The listing builds one solid part. Answer for the finished solid, in the listing's coordinates (mm). A direction names the side the tool comes from. Give positions to 0.01 mm unless a question says otherwise; leave off trailing zeros. Loops run counter-clockwise (first coordinate to the right, second up) from the corner with the lowest first, then second, coordinate; pieces in that order, holes last. Notation, with made-up numbers: M -4.5,74 L 0.5,74 A21 ccw 0.5,86 Z; hole C 30.25,-23.5 d4. An arc over 180 degrees is marked long. Return JSON: item names as keys, results as strings.
from build123d import *

# Parameters (mm, degrees)
SKETCH_1_W          = 400
SKETCH_1_H          = 350
EXTRUDE_1_DEPTH     = 80
SKETCH_2_W          = 394
SKETCH_2_H          = 344
EXTRUDE_2_DEPTH     = 10
SKETCH_3_W          = 388
SKETCH_3_H          = 338
CUT_EXTRUDE_1_DEPTH = 50
SKETCH_4_W          = 388
SKETCH_4_H          = 3
EXTRUDE_3_DEPTH     = 30
SKETCH_5_W          = 3
SKETCH_5_H          = 162
SKETCH_5_H_2        = 90
EXTRUDE_4_DEPTH     = 30
SKETCH_6_W          = 350
SKETCH_6_H          = 34
CUT_EXTRUDE_2_DEPTH = 320
CHAMFER_1_SIZE      = 20


with BuildPart() as part:
    # 草图1 → 凸台-拉伸1 (new body)
    with BuildSketch(Plane.XY):
        Rectangle(SKETCH_1_W, SKETCH_1_H)
    extrude(amount=EXTRUDE_1_DEPTH)

    # 草图2 → 凸台-拉伸2 (add)
    with BuildSketch(Plane.XY.offset(80)):
        Rectangle(SKETCH_2_W, SKETCH_2_H)
    extrude(amount=EXTRUDE_2_DEPTH)

    # 草图3 → 切除-拉伸1 (cut)
    with BuildSketch(Plane.XY.offset(90)):
        Rectangle(SKETCH_3_W, SKETCH_3_H)
    extrude(amount=-CUT_EXTRUDE_1_DEPTH, mode=Mode.SUBTRACT)

    # 草图4 → 凸台-拉伸3 (add)
    with BuildSketch(Plane.XY.offset(40)):
        with Locations((0, 87.5)):
            Rectangle(SKETCH_4_W, SKETCH_4_H)
        with Locations((0, -77.5)):
            Rectangle(SKETCH_4_W, SKETCH_4_H)
    extrude(amount=EXTRUDE_3_DEPTH)

    # 草图5 → 凸台-拉伸4 (add)
    with BuildSketch(Plane.XY.offset(40)):
        with Locations((-87.5, 5)):
            Rectangle(SKETCH_5_W, SKETCH_5_H)
        with Locations((-1.5, 5)):
            Rectangle(SKETCH_5_W, SKETCH_5_H)
        with Locations((142.5, 5)):
            Rectangle(SKETCH_5_W, SKETCH_5_H)
        with Locations((-122.5, -124)):
            Rectangle(SKETCH_5_W, SKETCH_5_H_2)
    extrude(amount=EXTRUDE_4_DEPTH)

    # 草图6 → 切除-拉伸2 (cut)
    with BuildSketch(Plane.XZ.offset(175)):
        with Locations((0, 20)):
            Rectangle(SKETCH_6_W, SKETCH_6_H)
    extrude(amount=-CUT_EXTRUDE_2_DEPTH, mode=Mode.SUBTRACT)

    # 倒角1
    chamfer_1_edges = [part.edges().sort_by_distance(p)[0] for p in [
        (175, -175, 20),
        (-175, -175, 20),
    ]]
    chamfer(chamfer_1_edges, length=CHAMFER_1_SIZE)


solid = part.part
(1) Determine the mould class of faces 1 (the flat face through (-200, -2, 39)), 2 (the flat face through (-89, 4, 55)), 3 (the flat face through (-3, 175, 39)) for opening direction X: released by +X, released by -X, zero draft, split by the parting line, or undercut.
Values follow:
{"face 1": "released by -X", "face 2": "undercut", "face 3": "zero draft"}
(2) The part is cut by section C-C (x = 94). Determine the outline of the cut face in (y, z), and give its area (3 significant figures).
Values follow:
{"outline": "M -175,0 L 175,0 L 175,80 L 172,80 L 172,90 L 169,90 L 169,40 L 89,40 L 89,70 L 86,70 L 86,40 L -76,40 L -76,70 L -79,70 L -79,40 L -169,40 L -169,90 L -172,90 L -172,80 L -175,80 L -175,37 L 145,37 L 145,3 L -175,3 Z", "area": "3,840 mm²"}
(3) A tool of negligible diameter and unlimited length cuts with its end or side. For faces 4 (the flat face through (185, -165, 20)), 5 (the flat face through (194, -2, 65)), from which of +Z, -Z, +X, -X, +Y, -Y can it reach the whole face along a straight path? Write none if from no direction.
Values follow:
{"face 4": "-Y", "face 5": "+Z"}
(4) The part is cut by section B-B (z = 32.5). Determine the outline of the cut face in (x, y), and give its area (3 significant figures).
Values follow:
{"outline": "M -200,-175 L -195,-175 L -175,-155 L -175,145 L 175,145 L 175,-155 L 195,-175 L 200,-175 L 200,175 L -200,175 Z", "area": "27,600 mm²"}
(5) The part is cut by section A-A (y = -132). Determine the outline of the cut face in (x, z).
Values follow:
{"outline": "M -200,0 L 200,0 L 200,80 L 197,80 L 197,90 L 194,90 L 194,40 L -121,40 L -121,70 L -124,70 L -124,40 L -194,40 L -194,90 L -197,90 L -197,80 L -200,80 Z; hole M -175,3 L 175,3 L 175,37 L -175,37 Z"}
(6) Given pin 1 (12 mm diameter, centred on x = -158.5, y = 34, fed in from +Z); pin 2 (10 mm diameter, centred on x = -26, z = 18.5, fed in from -Y); pin 3 (5 mm diameter, centred on y = -67, z = 85, fed in from -X), each flat-ended and moving along its own axis, determine where each tip first touches the part or whether it passes through.
Values follow:
{"pin 1": "z = 40", "pin 2": "y = 145", "pin 3": "x = -197"}
(7) Straight lines are drawn through the part: line 1 along Y through (x, z) = (94.5, 67); line 2 along X through (y, z) = (64.5, 34); line 3 along Z through (x, y) = (-11.5, -92.5). For each, find the intervals that lie inside material, in ascending order.
Values follow:
{"line 1": "-175 to -169, -79 to -76, 86 to 89, 169 to 175", "line 2": "-200 to -175, 175 to 200", "line 3": "0 to 3, 37 to 40"}
(8) The part is cut by section D-D (y = 25). Determine the outline of the cut face in (x, z).
Values follow:
{"outline": "M -200,0 L 200,0 L 200,80 L 197,80 L 197,90 L 194,90 L 194,40 L 144,40 L 144,70 L 141,70 L 141,40 L 0,40 L 0,70 L -3,70 L -3,40 L -86,40 L -86,70 L -89,70 L -89,40 L -194,40 L -194,90 L -197,90 L -197,80 L -200,80 Z; hole M -175,3 L 175,3 L 175,37 L -175,37 Z"}
